Can you work these out from the drawing? Everything is in mm from the part's minimum corner. A direction names the side the tool comes from. Round coordinates to 2 decimals unless told otherwise and drop trailing zeros. Write each loop counter-clockwise with the first axis right and the second up, starting at its lowest first coordinate (ties: lowest second). Pieces come first, ordered by that corner, then holes. Notation, with made-up numbers: (36, -3.5) - (79, -3.5) arc R22 ccw to (79, 21.5) - close; hole circle Ø3 at (28.25, 16.5). An arc over 180 degrees is marked (long way). One line per item, written item: value. Start each with the question number.
(1) I'm going to push flat-ended pins straight in: pin 1 Ø3 at (x, z) = (13, 11) entering from +Y; pin 2 Ø5 at (y, z) = (7.5, 7.5) entering from +X; pin 3 Ø2 at (x, z) = (25, 1) entering from -Y. Where does each tip first touch, or does it pass through?
(2) Thinking about a two-plate mould opening in Z: for the marked faces 1, 2, 3 and 4, which applies, +Z half, -Z half, draft (parallel to the pull), parting line (faces both ways), or undercut?
(3) I want a section at A-A on x = 54. List the corners of the cut face in (y, z) for me, plus the area to 3 significant figures.
(4) I want a section at B-B on z = 7.5. List the corners of the cut face in (x, y) for me, plus the area to 3 significant figures.
(5) I want a section at C-C on y = 58. List the corners of the cut face in (x, z) for me.
(6) If I drill on L1, parallel to Y at x = 36, z = 10.5; L2, parallel to Z at x = 28, y = 35; L3, parallel to X at y = 44.5, z = 2, over which ranges is the centre line in solid material (lowest first)? Write a range as from..to.
(7) I want a section at D-D on z = 1.5. List the corners of the cut face in (x, y) for me, plus the area to 3 significant figures.
(8) On a 3-axis mill with a long thin cutter (end or side, diameter ignored), from which of +Z, -Z, +X, -X, +Y, -Y can I reach the whole of each face in a straight line? I mean the marked faces 5, 6 and 7. Say none if no direction works.
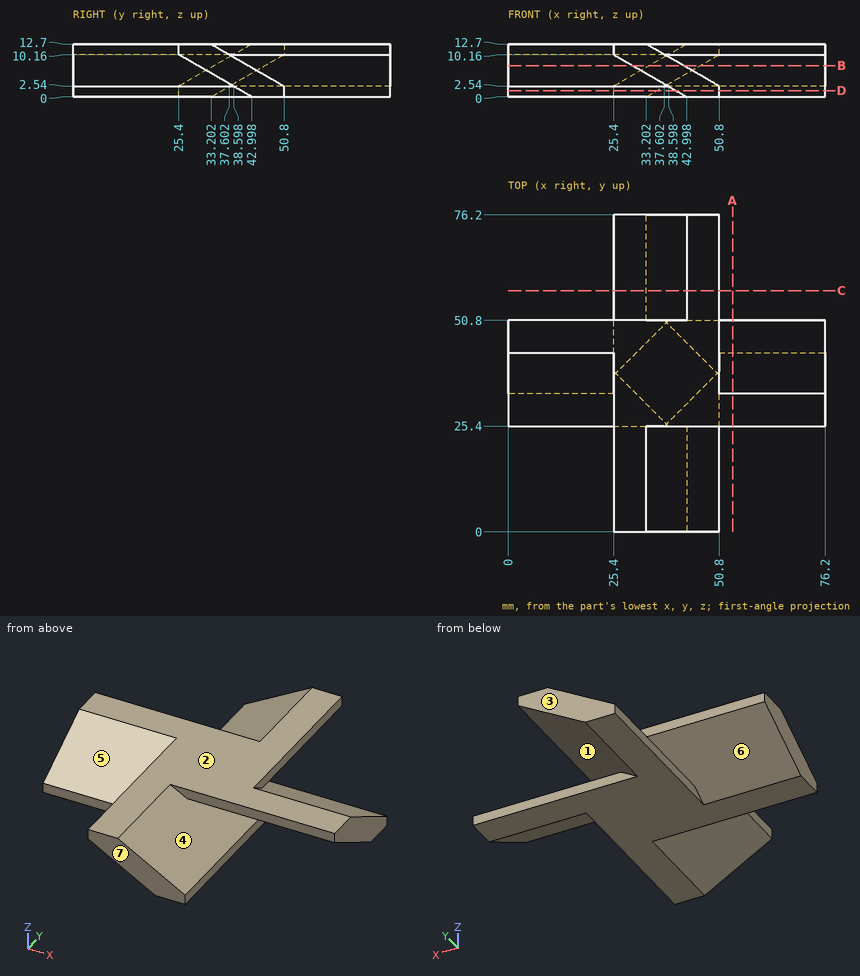
Established:
1. pin 1: y = 50.8
1. pin 2: x = 46.54
1. pin 3: y = 25.4
2. face 1: undercut
2. face 2: +Z half
2. face 3: draft
2. face 4: undercut
3. outline: (25.4, 10.16) - (43, 0) - (50.8, 0) - (50.8, 2.54) - (33.2, 12.7) - (25.4, 12.7) - close
3. area: 144 mm2
4. outline: (0, 33.99) - (30.01, 33.99) - (30.01, 0) - (42.21, 0) - (42.21, 30.01) - (76.2, 30.01) - (76.2, 42.21) - (46.19, 42.21) - (46.19, 76.2) - (33.99, 76.2) - (33.99, 46.19) - (0, 46.19) - close
4. area: 1,730 mm2
5. outline: (25.4, 0) - (33.2, 0) - (50.8, 10.16) - (50.8, 12.7) - (43, 12.7) - (25.4, 2.54) - close
6. L1: 0..50.8
6. L2: 0..8.08, 8.66..12.7
6. L3: 25.4..76.2
7. outline: (0, 25.4) - (40.4, 25.4) - (40.4, 0) - (50.8, 0) - (50.8, 40.4) - (76.2, 40.4) - (76.2, 50.8) - (35.8, 50.8) - (35.8, 76.2) - (25.4, 76.2) - (25.4, 35.8) - (0, 35.8) - close
7. area: 1,700 mm2
8. face 5: -X, -Y
8. face 6: -X, +Y
8. face 7: +Z, -Z, +X, -X, -Y
